from build123d import *

# Parameters (mm, degrees)
F0_R     = 63.5
F1_DEPTH = 85.598
F2_T     = -2.54
F3_R     = 9.5217645964
F4_DEPTH = 92.964


# Not quite as in the source:
# - a fillet or chamfer that OpenCascade refuses, or shapes differently, is made with other operations: its cross-section is extruded or revolved along the edge and cut away or added


with BuildPart() as f1:
    # F0 (on Top) → F1 (new body)
    with BuildSketch(Plane.XY):
        Circle(F0_R)
    extrude(amount=F1_DEPTH)

    # F2
    f2_openings = [f1.faces().sort_by_distance(p)[0] for p in [
        (0, 0, 85.598),
        (0, 0, 0),
    ]]
    offset(amount=F2_T, openings=f2_openings)

    # F3 (on Front) → F4 (cut, symmetric)
    with BuildSketch(Plane.XZ):
        with Locations((0, 41.1053188145)):
            Circle(F3_R)
    extrude(amount=F4_DEPTH, both=True, mode=Mode.SUBTRACT)

    # F5: fillet of radius 5.08 on 2 edges, made by hand

    # F5_s1 → F5_t2 (revolve, cut)
    with BuildSketch(Plane.XZ):
        with BuildLine():
            ThreePointArc((63.5, 81.1985909488), (62.8194090512, 83.7385909488), (60.96, 85.598))
            Line((60.96, 85.598), (63.5, 85.598))
            Line((63.5, 85.598), (63.5, 81.1985909488))
        make_face()
    revolve(axis=Axis((0, 0, 85.598), (0, 0, 1)), mode=Mode.SUBTRACT)

    # F5_s3 → F5_t4 (revolve, cut)
    with BuildSketch(Plane.XZ):
        with BuildLine():
            ThreePointArc((63.5, 4.3994090512), (62.8194090512, 1.8594090512), (60.96, 0))
            Line((60.96, 0), (63.5, 0))
            Line((63.5, 0), (63.5, 4.3994090512))
        make_face()
    revolve(axis=Axis((0, 0, 0), (0, 0, 1)), mode=Mode.SUBTRACT)


solid = f1.part
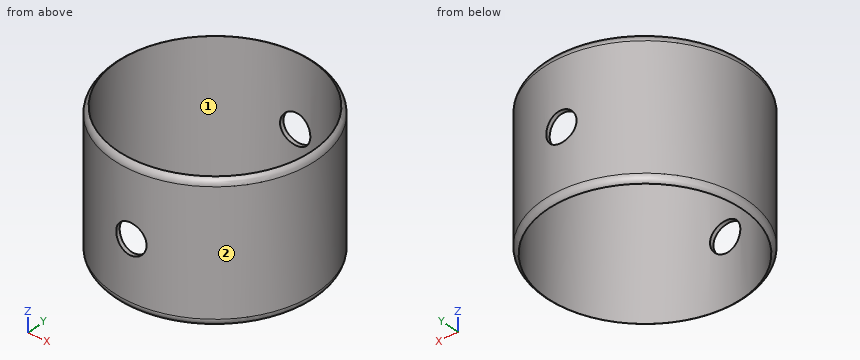
Geometry check sheet. Reference: the model listing, model coordinates, mm. Face numbers are marked on the shaded views. Round coordinates to 2 decimals unless told otherwise and drop trailing zeros. Write each loop counter-clockwise with the first axis right and the second up, starting at its lowest first coordinate (ties: lowest second). Pieces come first, ordered by that corner, then holes. Notation, with made-up numbers: (-32, 28) - (-3, 28) arc R23 ccw to (-3, 43) - close; hole circle Ø8 at (71.5, 14). An arc over 180 degrees is marked (long way). One line per item, written item: value.
1. Cross-section at B-B on x = 0. Record the boundary of the cut face in (y, z), and give its area (3 significant figures).
The answers:
outline: (-63.5, 4.4) arc R5.08 ccw to (-60.96, 0) - (-60.96, 31.58) - (-63.5, 31.58) - close; (-63.5, 50.63) - (-60.96, 50.63) - (-60.96, 85.6) arc R5.08 ccw to (-63.5, 81.2) - close; (60.96, 0) arc R5.08 ccw to (63.5, 4.4) - (63.5, 31.58) - (60.96, 31.58) - close; (60.96, 50.63) - (63.5, 50.63) - (63.5, 81.2) arc R5.08 ccw to (60.96, 85.6) - close
area: 325 mm^2
2. Mould release check, pull along X, two halves, no side actions. Record for the marked faces 1 and 2: released by +X, released by -X, zero draft, split by the parting line, or undercut.
The answers:
face 1: undercut
face 2: split by the parting line
3. Cross-section at A-A on y = 0. Record the boundary of the cut face in (x, z), and give its area (3 significant figures).
The answers:
outline: (-63.5, 4.4) arc R5.08 ccw to (-60.96, 0) - (-60.96, 85.6) arc R5.08 ccw to (-63.5, 81.2) - close; (60.96, 0) arc R5.08 ccw to (63.5, 4.4) - (63.5, 81.2) arc R5.08 ccw to (60.96, 85.6) - close
area: 422 mm^2
4. Scan lines: L1, parallel to Y at x = 0, z = 64.5; L2, parallel to Y at x = -40, z = 74.5; L3, parallel to X at y = 20.5, z = 51. Record each from-to range of solid material in increasing order.
The answers:
L1: y = -63.5 to -60.96, 60.96 to 63.5
L2: y = -49.32 to -46, 46 to 49.32
L3: x = -60.1 to -57.41, 57.41 to 60.1
5. Cross-section at C-C on z = 69.5. Record the boundary of the cut face in (x, y).
The answers:
outline: circle Ø127 at (0, 0); hole circle Ø121.92 at (0, 0)
6. Depth check by flat-ended pin: pin 1 Ø5 at (x, z) = (40.5, 30.5) entering from -Y; pin 2 Ø1.5 at (x, z) = (21.5, 15.5) entering from +Y; pin 3 Ø3 at (y, z) = (32, 41.5) entering from -X. Enter the tip coordinate at first touch or a pass-through.
The answers:
pin 1: stops at y = -50.87
pin 2: stops at y = 60.01
pin 3: stops at x = -55.7
